```python
from build123d import *

# Parameters (mm, degrees)
SKETCH2_R           = 1.5
BOSS_EXTRUDE1_DEPTH = 15
CHAMFER1_SIZE       = 0.3
SKETCH6_W           = 3
SKETCH6_H           = 2.75
CUT_EXTRUDE1_DEPTH  = 1.6
SKETCH8_R           = 1.493375673
CUT_EXTRUDE2_DEPTH  = 1
CUT_EXTRUDE2_TAPER  = 45


with BuildPart() as part:
    # Sketch2 → Boss-Extrude1 (new body)
    with BuildSketch(Plane(origin=(0, 0, 0), x_dir=(0, 0, -1), z_dir=(1, 0, 0))):
        Circle(SKETCH2_R)
    extrude(amount=-BOSS_EXTRUDE1_DEPTH)

    # Chamfer1
    chamfer1_edges = [part.edges().sort_by_distance(p)[0] for p in [
        (0, 0, 1.5),
    ]]
    chamfer(chamfer1_edges, length=CHAMFER1_SIZE)

    # Sketch6 → Revolve1 (revolve)
    with BuildSketch(Plane.XY):
        with Locations((-16.5, 1.375)):
            Rectangle(SKETCH6_W, SKETCH6_H)
    revolve(axis=Axis((-15, 0, 0), (1, 0, 0)))

    # Sketch7 → Cut-Extrude1 (cut)
    with BuildSketch(Plane.ZY.offset(18)):
        Polygon((0, 1.443375673), (-1.25, 0.721687836), (-1.25, -0.721687836), (0, -1.443375673), (1.25, -0.721687836), (1.25, 0.721687836), align=None)
    extrude(amount=-CUT_EXTRUDE1_DEPTH, mode=Mode.SUBTRACT)

    # Sketch8 → Cut-Extrude2 (cut)
    with BuildSketch(Plane.ZY.offset(18)):
        Circle(SKETCH8_R)
    extrude(amount=-CUT_EXTRUDE2_DEPTH, taper=CUT_EXTRUDE2_TAPER, mode=Mode.SUBTRACT)


solid = part.part
```
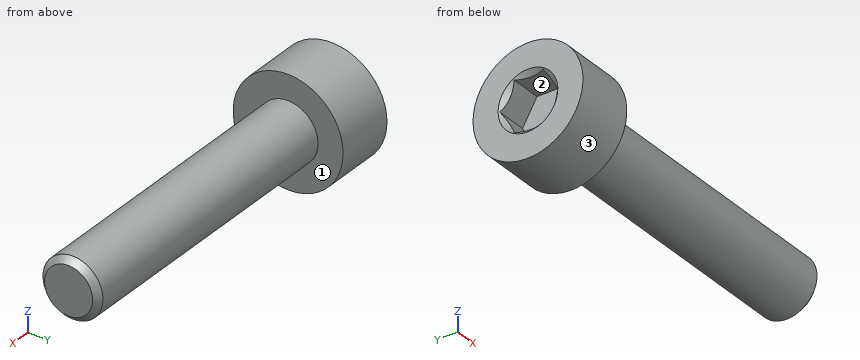
The model under review builds one solid part; all positions refer to its coordinate system, in mm. Face numbers are marked on the shaded views. A direction names the side the tool comes from. Round coordinates to 2 decimals unless told otherwise and drop trailing zeros. Write each loop counter-clockwise with the first axis right and the second up, starting at its lowest first coordinate (ties: lowest second). Pieces come first, ordered by that corner, then holes.
(1) We need section C-C on y = 2.05. Give the boundary of the cut face in (x, z), and give its area (3 significant figures).
(2) We need section B-B on z = -2.2. Give the boundary of the cut face in (x, y).
(3) Machinability: for the marked faces 1, 2 and 3, which of the approach directions +Z, -Z, +X, -X, +Y, -Y give a long, thin tool a straight path to every point of the face, cutting with its end or side? Answer none if there is none.
(4) We need section A-A on x = -14. Give the boundary of the cut face in (y, z).
(5) Wall thickness on L1, parallel to X at y = 1.2, z = 1.15; L2, parallel to X at y = 0.05, z = -0.7; L3, parallel to Y at x = -11, z = 0.9: over which ranges is each line inside the solid? List them lowest first.
(6) Insertion check: pin 1 (3 mm diameter, centred on y = 0.5, z = 0.5, fed in from -X); pin 2 (2 mm diameter, centred on x = -13, z = 1.5, fed in from -Y); pin 3 (0.8 mm diameter, centred on y = 0, z = 0.5, fed in from -X); pin 4 (2 mm diameter, centred on x = -15.5, y = 1.5, fed in from +Z). Each pin has a flat end and moves straight along its axis. Give the tip position at first contact, or say it passes through.
Findings below:
1. outline: (-18, -1.83) - (-15, -1.83) - (-15, 1.83) - (-18, 1.83) - close
1. area: 11.0 mm2
2. outline: (-18, -1.65) - (-15, -1.65) - (-15, 1.65) - (-18, 1.65) - close
3. face 1: +X
3. face 2: -X
3. face 3: +X, -X
4. outline: circle Ø3 at (0, 0)
5. L1: x = -18 to -15
5. L2: x = -16.4 to 0
5. L3: y = -1.2 to 1.2
6. pin 1: stops at x = -18
6. pin 2: stops at y = -1.41
6. pin 3: stops at x = -16.4
6. pin 4: stops at z = 2.7
